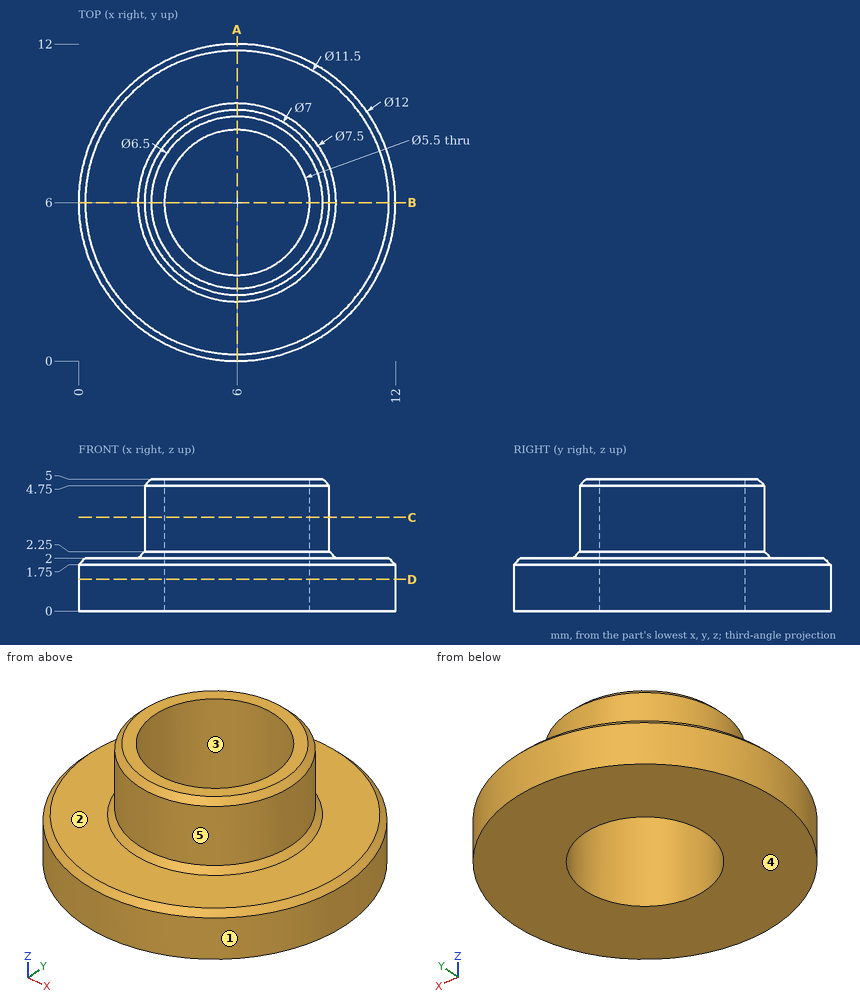
For this review, use the dimensioned drawing (mm, ordinates from the lowest corner) and the shaded views. A direction names the side the tool comes from. Round coordinates to 2 decimals unless told otherwise and drop trailing zeros. Write each loop counter-clockwise with the first axis right and the second up, starting at its lowest first coordinate (ties: lowest second). Pieces come first, ordered by that corner, then holes. Notation, with made-up numbers: (14, 31.25) -> (36, 31.25) arc R10 cw to (36, 37.25) -> close; hole circle Ø3 at (14, -4.5). An arc over 180 degrees is marked (long way). Answer in a Markdown table with one row per item.
Q1. For the marked faces 4 and 5, list the 3-axis set-ups (+Z, -Z, +X, -X, +Y, -Y) from which the entire face can be reached by the end or side of a thin tool; tool diameter is ignored.
The answers:
| item | result |
|---|---|
| face 4 | -Z, +X, -X, +Y, -Y |
| face 5 | +Z |
Q2. Take a section at D-D, the plane z = 1.2. State the section outline as (x, y) points.
The answers:
| item | result |
|---|---|
| outline | circle Ø12 at (6, 6); hole circle Ø5.5 at (6, 6) |
Q3. Clearance check with flat-ended pins moving along their axes: pin 1 Ø3 at (y, z) = (1.5, 4.5) entering from -X; pin 2 Ø6 at (x, y) = (1.5, 6) entering from +Z. State where each tip first meets the part, or that it passes through.
The answers:
| item | result |
|---|---|
| pin 1 | x = 4.2 |
| pin 2 | z = 5 |
Q4. Take a section at C-C, the plane z = 3.55. State the section outline as (x, y) points.
The answers:
| item | result |
|---|---|
| outline | circle Ø7 at (6, 6); hole circle Ø5.5 at (6, 6) |
Q5. Take a section at A-A, the plane x = 6. State the section outline as (y, z) points.
The answers:
| item | result |
|---|---|
| outline | (0, 0) -> (3.25, 0) -> (3.25, 5) -> (2.75, 5) -> (2.5, 4.75) -> (2.5, 2.25) -> (2.25, 2) -> (0.25, 2) -> (0, 1.75) -> close; (8.75, 0) -> (12, 0) -> (12, 1.75) -> (11.75, 2) -> (9.75, 2) -> (9.5, 2.25) -> (9.5, 4.75) -> (9.25, 5) -> (8.75, 5) -> close |
Q6. To check wall thickness, follow L1, parallel to Y at x = 6, z = 3.9; L2, parallel to Y at x = 6, z = 1.35; L3, parallel to Z at x = 10, y = 5. State the ranges of each line that lie inside material, in increasing order. Write a range as [from, to].
The answers:
| item | result |
|---|---|
| L1 | [2.5, 3.25], [8.75, 9.5] |
| L2 | [0, 3.25], [8.75, 12] |
| L3 | [0, 2] |
Q7. Draft analysis for pull direction Y (two halves, no side actions). For the marked faces 1, 2 and 3, state which applies: +Y half, -Y half, draft (parallel to the pull), parting line (faces both ways), or undercut.
The answers:
| item | result |
|---|---|
| face 1 | parting line |
| face 2 | draft |
| face 3 | undercut |
